Verification items for the finished model (mm, model axes). A direction names the side the tool comes from. Round coordinates to 2 decimals unless told otherwise and drop trailing zeros. Loops run counter-clockwise (first coordinate to the right, second up) from the corner with the lowest first, then second, coordinate; pieces in that order, holes last. Notation, with made-up numbers: M 33.25,87 L 80.25,87 A13 ccw 80.25,98 Z; hole C 43.25,80.5 d2. An arc over 180 degrees is marked long. One line per item, written item: value.
from build123d import *

# Parameters (mm, degrees)
EXTRUDE_1_DEPTH             = 700
SKETCH_2_R                  = 2.25
CUT_EXTRUDE_1_DEPTH         = 10
SKETCH_3_R                  = 4
CUT_EXTRUDE_2_DEPTH         = 51
HOLE_WIZARD_3_5_3_5_1_D     = 3.5
HOLE_WIZARD_3_5_3_5_1_DEPTH = 2
HOLE_WIZARD_3_5_3_5_1_TIP   = 1.051506083


with BuildPart() as part:
    # 草圖1 → 填料-伸長1 (new body)
    with BuildSketch(Plane.XY):
        Polygon((0, 50), (0, 0), (50, 0), (50, 1.8), (1.8, 1.8), (1.8, 50), align=None)
    extrude(amount=EXTRUDE_1_DEPTH)

    # 草圖2 → 除料-伸長1 (cut)
    with BuildSketch(Plane(origin=(0, 0, 0), x_dir=(-1, 0, 0), z_dir=(0, -1, 0))):
        with Locations((-38.5, -20)):
            Circle(SKETCH_2_R)
        with Locations((-38.5, -58.34)):
            Circle(SKETCH_2_R)
        with Locations((-11.5, -20)):
            Circle(SKETCH_2_R)
        with Locations((-11.5, -58.34)):
            Circle(SKETCH_2_R)
    extrude(amount=-CUT_EXTRUDE_1_DEPTH, mode=Mode.SUBTRACT)

    # 草圖3 → 除料-伸長2 (cut, through all)
    with BuildSketch(Plane.ZY):
        with Locations((600, 20)):
            Circle(SKETCH_3_R)
        with Locations((500, 20)):
            Circle(SKETCH_3_R)
        with Locations((400, 20)):
            Circle(SKETCH_3_R)
        with Locations((300, 20)):
            Circle(SKETCH_3_R)
    extrude(amount=-CUT_EXTRUDE_2_DEPTH, mode=Mode.SUBTRACT)

    # Ø3.5 (3.5) 直徑孔1
    with Locations(Plane(origin=(0, 0, 0), x_dir=(-1, 0, 0), z_dir=(0, -1, 0))):
        with Locations((-13.5, -685), (-13.5, -675), (-13.5, -625), (-13.5, -255), (-13.5, -265), (-13.5, -315)):
            Hole(HOLE_WIZARD_3_5_3_5_1_D / 2, depth=HOLE_WIZARD_3_5_3_5_1_DEPTH)
            with Locations((0, 0, -(HOLE_WIZARD_3_5_3_5_1_DEPTH + HOLE_WIZARD_3_5_3_5_1_TIP / 2))):  # 118° drill point
                Cone(0, HOLE_WIZARD_3_5_3_5_1_D / 2, HOLE_WIZARD_3_5_3_5_1_TIP, mode=Mode.SUBTRACT)


solid = part.part
(1) Depth check by flat-ended pin: pin 1 Ø4.5 at (x, z) = (13.5, 265) entering from +Y; pin 2 Ø13 at (y, z) = (20, 400) entering from +X; pin 3 Ø4 at (x, z) = (38.5, 20) entering from +Y. Enter the tip coordinate at first touch or a pass-through.
Completed:
pin 1: stops at y = 1.8
pin 2: stops at x = 1.8
pin 3: passes through
(2) Thickness scan on L1, parallel to Z at x = 38.5, y = 1.3; L2, parallel to X at y = 1.25, z = 625; L3, parallel to Y at x = 46.5, z = 567.5. Record the ranges inside material, lowest first. Write a range as from..to.
Completed:
L1: z = 0..17.75, 22.25..56.09, 60.59..700
L2: x = 0..11.75, 15.25..50
L3: y = 0..1.8
(3) Sectioned sample at B-B on x = 30.5. Enter the section's corners in (y, z).
Completed:
outline: M 0,0 L 1.8,0 L 1.8,700 L 0,700 Z
(4) Tool access check on faces 1 (the face through (1.8, 26, 345)), 2 (the face through (0, 25, 345)). Record the directions out of +Z, -Z, +X, -X, +Y, -Y that give a thin tool (end or side, any length) a straight path to the whole face; none if there is none.
Completed:
face 1: +Z, -Z, +X, +Y
face 2: +Z, -Z, -X, +Y, -Y
(5) Sectioned sample at A-A on z = 241. Enter the section's corners in (x, y), and give its area (3 significant figures).
Completed:
outline: M 0,0 L 50,0 L 50,1.8 L 1.8,1.8 L 1.8,50 L 0,50 Z
area: 177 mm^2
